from build123d import *

# Parameters (mm, degrees)
SKETCH1_W               = 120
SKETCH1_H               = 74.5
BOSS_EXTRUDE1_DEPTH     = 2
SKETCH2_W               = 120
SKETCH2_H               = 69
BOSS_EXTRUDE2_DEPTH     = 3
SKETCH3_W               = 40.5
SKETCH3_H               = 55.5
SKETCH3_W_2             = 28.5
SKETCH3_H_2             = 43.5
BOSS_EXTRUDE3_DEPTH     = 16
SKETCH4_W               = 25
SKETCH4_H               = 14.5
CUT_EXTRUDE1_DEPTH      = 16
CUT_EXTRUDE2_DEPTH      = 16
SKETCH6_R               = 1.5
CUT_EXTRUDE3_DEPTH      = 10
SKETCH7_R               = 10
CUT_EXTRUDE4_DEPTH      = 17
CUT_EXTRUDE4_DEPTH_BACK = 6


with BuildPart() as part:
    # Sketch1 → Boss-Extrude1 (new body)
    with BuildSketch(Plane(origin=(0, 0, 0), x_dir=(1, 0, 0), z_dir=(0, 1, 0))):
        Rectangle(SKETCH1_W, SKETCH1_H)
    extrude(amount=BOSS_EXTRUDE1_DEPTH)

    # Sketch2 → Boss-Extrude2 (add)
    with BuildSketch(Plane(origin=(0, 2, 0), x_dir=(1, 0, 0), z_dir=(0, 1, 0))):
        Rectangle(SKETCH2_W, SKETCH2_H)
    extrude(amount=BOSS_EXTRUDE2_DEPTH)

    # Sketch3 → Boss-Extrude3 (add)
    with BuildSketch(Plane(origin=(0, 5, 0), x_dir=(1, 0, 0), z_dir=(0, 1, 0))):
        with Locations((0, 0.5)):
            Rectangle(SKETCH3_W, SKETCH3_H)
        with Locations((0, 0.5)):
            Rectangle(SKETCH3_W_2, SKETCH3_H_2, mode=Mode.SUBTRACT)
    extrude(amount=BOSS_EXTRUDE3_DEPTH)

    # Sketch4 → Cut-Extrude1 (cut)
    with BuildSketch(Plane.XY.offset(27.25)):
        with Locations((0.25, 13.75)):
            Rectangle(SKETCH4_W, SKETCH4_H)
    extrude(amount=-CUT_EXTRUDE1_DEPTH, mode=Mode.SUBTRACT)

    # Sketch5 → Cut-Extrude2 (cut)
    with BuildSketch(Plane(origin=(0, 0, -28.25), x_dir=(-1, 0, 0), z_dir=(0, 0, -1))):
        with BuildLine():
            Line((-7.05, 21), (-11.25, 21))
            Line((-11.25, 21), (-11.25, 12.75))
            ThreePointArc((-11.25, 12.75), (-9.15, 14.85), (-7.05, 12.75))
            Line((-7.05, 12.75), (-7.05, 21))
        make_face()
        with BuildLine():
            ThreePointArc((-7.05, 12.75), (-9.15, 14.85), (-11.25, 12.75))
            Line((-11.25, 12.75), (-7.05, 12.75))
        make_face()
        with BuildLine():
            Line((-7.05, 12.75), (-11.25, 12.75))
            ThreePointArc((-11.25, 12.75), (-9.15, 10.65), (-7.05, 12.75))
        make_face()
        with BuildLine():
            ThreePointArc((11.25, 12.75), (9.15, 14.85), (7.05, 12.75))
            Line((7.05, 12.75), (11.25, 12.75))
        make_face()
        with BuildLine():
            Line((11.25, 12.75), (7.05, 12.75))
            ThreePointArc((7.05, 12.75), (9.15, 10.65), (11.25, 12.75))
        make_face()
        with BuildLine():
            Line((11.25, 21), (7.05, 21))
            Line((7.05, 21), (7.05, 12.75))
            ThreePointArc((7.05, 12.75), (9.15, 14.85), (11.25, 12.75))
            Line((11.25, 12.75), (11.25, 21))
        make_face()
    extrude(amount=-CUT_EXTRUDE2_DEPTH, mode=Mode.SUBTRACT)

    # Sketch6 → Cut-Extrude3 (cut)
    with BuildSketch(Plane(origin=(0, 21, 0), x_dir=(1, 0, 0), z_dir=(0, 1, 0))):
        with Locations((17.25, 25.25)):
            Circle(SKETCH6_R)
        with Locations((17.25, -24.25)):
            Circle(SKETCH6_R)
        with Locations((-17.25, -24.25)):
            Circle(SKETCH6_R)
        with Locations((-17.25, 25.25)):
            Circle(SKETCH6_R)
    extrude(amount=-CUT_EXTRUDE3_DEPTH, mode=Mode.SUBTRACT)

    # Sketch7 → Cut-Extrude4 (cut, two sides)
    with BuildSketch(Plane(origin=(0, 5, 0), x_dir=(1, 0, 0), z_dir=(0, 1, 0))) as cut_extrude4_sk:
        with Locations((-40, 0)):
            Circle(SKETCH7_R)
        with Locations((40, 0)):
            Circle(SKETCH7_R)
    extrude(amount=CUT_EXTRUDE4_DEPTH, mode=Mode.SUBTRACT)
    extrude(cut_extrude4_sk.sketch, amount=-CUT_EXTRUDE4_DEPTH_BACK, mode=Mode.SUBTRACT)


solid = part.part
CAD build for the part. Positions are in the model's coordinates, mm. A direction names the side the tool comes from. Round coordinates to 2 decimals unless told otherwise and drop trailing zeros. Write each loop counter-clockwise with the first axis right and the second up, starting at its lowest first coordinate (ties: lowest second). Pieces come first, ordered by that corner, then holes.
(1) Drop flat-ended pins along their axis: P1, Ø1.5, axis at x = 10, y = 9.5, coming from the -Z side; P2, Ø8.5, axis at x = 3, z = 0.5, coming from the +Y side; P3, Ø1.5, axis at x = 24.5, y = 3.5, coming from the -Z side; P4, Ø12, axis at x = -4, z = -10.5, coming from the -Y side. Give the stop position or say it passes through.
(2) Slice it at A-A, the plane z = -6. Write the cut outline in (x, y), and give its area (3 significant figures).
(3) Slice it at B-B, the plane x = 40. Write the cut outline in (y, z).
(4) 3-axis set-ups, long thin cutter, end or side, ignore diameter. For faces 1 (the face through (-20.25, 13, 0)), 2 (the face through (-1, 2, -36)), 3 (the face through (-11.25, 17, -25)), 4 (the face through (-2, 6, 21.25)), 5 (the face through (-1, 2, 36)): which of +Z, -Z, +X, -X, +Y, -Y reach the whole face in a straight line?
(5) Mould opens along X. For faces 6 (the face through (17, 21, -1)), 7 (the face through (7.05, 17, -25)), 8 (the face through (20.25, 13, 0)) say: pulls with the +X half, pulls with the -X half, needs draft (parallel to the pull), parting line crosses it, or undercut.
(6) Slice it at C-C, the plane x = 17.25. Write the cut outline in (y, z).
(7) Slice it at D-D, the plane z = -20. Write the cut outline in (x, y).
(8) Probe line 1 along X through (y, z) = (17, -25.25); line 2 along Z through (x, y) = (-17.25, 17); line 3 along X through (y, z) = (19.25, 24.25). List the from-to ranges inside material, lowest first.
From the geometry:
1. P1: stops at z = -28.25
1. P2: stops at y = 5
1. P3: stops at z = -34.5
1. P4: stops at y = 0
2. outline: (-60, 0) - (-48, 0) - (-48, 5) - (-60, 5) - close; (-32, 0) - (32, 0) - (32, 5) - (20.25, 5) - (20.25, 21) - (14.25, 21) - (14.25, 5) - (-14.25, 5) - (-14.25, 21) - (-20.25, 21) - (-20.25, 5) - (-32, 5) - close; (48, 0) - (60, 0) - (60, 5) - (48, 5) - close
2. area: 632 mm2
3. outline: (0, -37.25) - (2, -37.25) - (2, -34.5) - (5, -34.5) - (5, -10) - (0, -10) - close; (0, 10) - (5, 10) - (5, 34.5) - (2, 34.5) - (2, 37.25) - (0, 37.25) - close
4. face 1: +Z, -Z, -X, +Y
4. face 2: -Z, +X, -X, +Y
4. face 3: +Z, -Z, +Y
4. face 4: +Y
4. face 5: +Z, +X, -X, +Y
5. face 6: needs draft
5. face 7: undercut
5. face 8: pulls with the +X half
6. outline: (0, -37.25) - (2, -37.25) - (2, -34.5) - (5, -34.5) - (5, -28.25) - (21, -28.25) - (21, -26.75) - (11, -26.75) - (11, -23.75) - (21, -23.75) - (21, 22.75) - (11, 22.75) - (11, 25.75) - (21, 25.75) - (21, 27.25) - (5, 27.25) - (5, 34.5) - (2, 34.5) - (2, 37.25) - (0, 37.25) - close
7. outline: (-60, 0) - (60, 0) - (60, 5) - (20.25, 5) - (20.25, 21) - (14.25, 21) - (14.25, 5) - (-14.25, 5) - (-14.25, 21) - (-20.25, 21) - (-20.25, 5) - (-60, 5) - close
8. line 1: x = -20.25 to -18.75, -15.75 to -11.25, -7.05 to 7.05, 11.25 to 15.75, 18.75 to 20.25
8. line 2: z = -28.25 to -26.75, -23.75 to 22.75, 25.75 to 27.25
8. line 3: x = -20.25 to -18.75, -15.75 to -12.25, 12.75 to 15.75, 18.75 to 20.25
